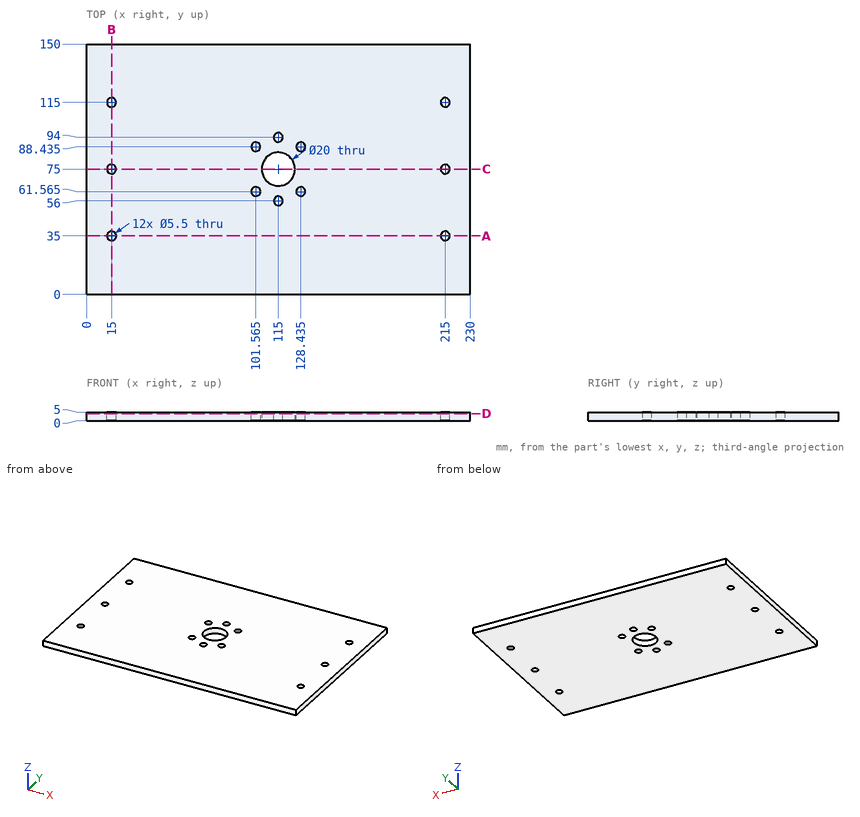
Drawing for the job (mm, zero at the part's lowest x, y, z). Give positions to 0.01 mm unless a question says otherwise; leave off trailing zeros. Loops run counter-clockwise (first coordinate to the right, second up) from the corner with the lowest first, then second, coordinate; pieces in that order, holes last.
1) Band-saw the part on C-C on y = 75. List the corners of the cut face in (x, z), then the cut area to 3 significant figures.
Values follow:
outline: (0, 0) - (12.25, 0) - (12.25, 5) - (0, 5) - close; (17.75, 0) - (105, 0) - (105, 5) - (17.75, 5) - close; (125, 0) - (212.25, 0) - (212.25, 5) - (125, 5) - close; (217.75, 0) - (230, 0) - (230, 5) - (217.75, 5) - close
area: 995 mm2
2) Band-saw the part on D-D on z = 4.15. State how many separate pieces and enclosed holes the cut face has, then the cut area to 3 significant figures.
Values follow:
separate pieces: 1
enclosed holes: 13
area: 33,900 mm2
3) Probe line 1 along Y through (x, z) = (215, 1.55); line 2 along Y through (x, z) = (115, 3.35); line 3 along X through (y, z) = (94.5, 0.3). List the from-to ranges inside material, lowest first.
Values follow:
line 1: y = 0 to 32.25, 37.75 to 72.25, 77.75 to 112.25, 117.75 to 150
line 2: y = 0 to 53.25, 58.75 to 65, 85 to 91.25, 96.75 to 150
line 3: x = 0 to 112.3, 117.7 to 230
4) Band-saw the part on A-A on y = 35. List the corners of the cut face in (x, z).
Values follow:
outline: (0, 0) - (12.25, 0) - (12.25, 5) - (0, 5) - close; (17.75, 0) - (212.25, 0) - (212.25, 5) - (17.75, 5) - close; (217.75, 0) - (230, 0) - (230, 5) - (217.75, 5) - close
5) Band-saw the part on B-B on x = 15. List the corners of the cut face in (y, z), then the cut area to 4 significant figures.
Values follow:
outline: (0, 0) - (32.25, 0) - (32.25, 5) - (0, 5) - close; (37.75, 0) - (72.25, 0) - (72.25, 5) - (37.75, 5) - close; (77.75, 0) - (112.25, 0) - (112.25, 5) - (77.75, 5) - close; (117.75, 0) - (150, 0) - (150, 5) - (117.75, 5) - close
area: 667.5 mm2
6) Drop a flat-ended pin along its axis: P1, Ø3.5, axis at x = 215, y = 75, coming from the +Z side. Give the stop position or say it passes through.
Values follow:
P1: passes through
